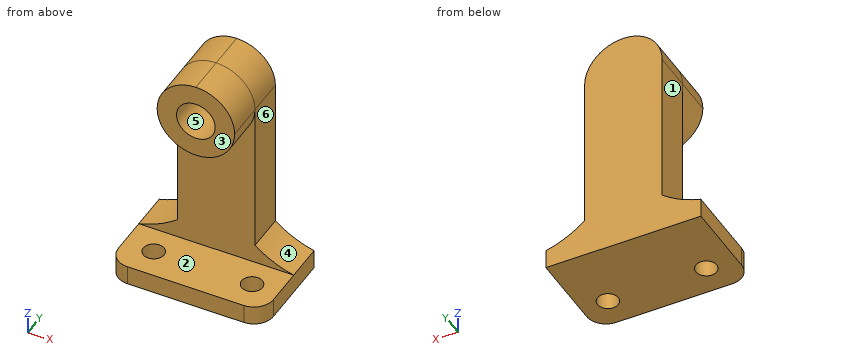
from build123d import *

# Parameters (mm, degrees)
F0_W      = 50.8
F0_H      = 76.2
F1_DEPTH  = 31.75
F2_W      = 19.05
F2_H      = 69.85
F3_DEPTH  = 50.8
F5_DEPTH  = 25.4
F6_R      = 6.35
F7_DEPTH  = 12.7
F8_DEPTH  = 25.4
F9_R      = 3.4236002905
F10_DEPTH = 25.4


with BuildPart() as f1:
    # F0 (on Front) → F1 (new body)
    with BuildSketch(Plane.XZ):
        with Locations((-25.4, 14.5882895922)):
            Rectangle(F0_W, F0_H)
    extrude(amount=F1_DEPTH)

    # F2 (on face) → F3 (cut)
    with BuildSketch(Plane.YZ):
        with Locations((-22.225, 17.7632895922)):
            Rectangle(F2_W, F2_H)
    extrude(amount=-F3_DEPTH, mode=Mode.SUBTRACT)

    # F4 (on face) → F5 (cut)
    with BuildSketch(Plane.XZ.offset(12.7)):
        with BuildLine():
            Line((-50.8, 52.6882895922), (-50.8, -17.1617104078))
            ThreePointArc((-50.8, -17.1617104078), (-44.1071699177, -14.6723705724), (-38.1, -10.8117104078))
            Line((-38.1, -10.8117104078), (-38.1, 52.6882895922))
            Line((-38.1, 52.6882895922), (-50.8, 52.6882895922))
        make_face()
        with BuildLine():
            Line((-12.7, 52.6882895922), (-12.7, -10.8117104078))
            ThreePointArc((-12.7, -10.8117104078), (-6.7122595502, -14.7112295081), (0, -17.1617104078))
            Line((0, -17.1617104078), (0, 52.6882895922))
            Line((0, 52.6882895922), (-12.7, 52.6882895922))
        make_face()
    extrude(amount=-F5_DEPTH, mode=Mode.SUBTRACT)

    # F6 (on face) → F7 (join)
    with BuildSketch(Plane.XZ.offset(12.7)):
        with BuildLine():
            ThreePointArc((-38.1, 39.9882895922), (-25.4, 27.2882895922), (-12.7, 39.9882895922))
            ThreePointArc((-12.7, 39.9882895922), (-16.4197438789, 48.9685457133), (-25.4, 52.6882895922))
            ThreePointArc((-25.4, 52.6882895922), (-34.3802561211, 48.9685457133), (-38.1, 39.9882895922))
        make_face()
        with Locations((-25.4, 39.9882895922)):
            Circle(F6_R, mode=Mode.SUBTRACT)
    extrude(amount=F7_DEPTH)

    # F8 (cut): faces of the model
    f8_faces = [f1.faces().sort_by_distance(p)[0] for p in [
        (-35.2632271754, -12.7, 49.8515167676),
        (-15.5367728246, -12.7, 49.8515167676),
    ]]
    extrude(f8_faces, amount=-F8_DEPTH, mode=Mode.SUBTRACT)

    # F9 (on face) → F10 (cut)
    with BuildSketch(Plane.XY.offset(-17.1617104078)):
        with Locations((-41.0295619067, -21.9763997095)):
            Circle(F9_R)
        with Locations((-8.7823613257, -21.9763997095)):
            Circle(F9_R)
        with BuildLine():
            Line((-50.8, -31.75), (-44.45, -31.75))
            ThreePointArc((-44.45, -31.75), (-48.9401280605, -29.8901280605), (-50.8, -25.4))
            Line((-50.8, -25.4), (-50.8, -31.75))
        make_face()
        with BuildLine():
            ThreePointArc((0, -25.4), (-1.8598719395, -29.8901280605), (-6.35, -31.75))
            Line((-6.35, -31.75), (0, -31.75))
            Line((0, -31.75), (0, -25.4))
        make_face()
    extrude(amount=-F10_DEPTH, mode=Mode.SUBTRACT)


solid = f1.part
Read the model definition and answer for the solid it produces. Units are mm, in the model's axes. Face numbers are marked on the shaded views. A direction names the side the tool comes from. Round coordinates to 2 decimals unless told otherwise and drop trailing zeros. Write each loop counter-clockwise with the first axis right and the second up, starting at its lowest first coordinate (ties: lowest second). Pieces come first, ordered by that corner, then holes.
Q1. Find section C-C on x = -23.5. Determine the outline of the cut face in (y, z), and give its area (3 significant figures).
Values:
outline: (-31.75, -23.51) - (0, -23.51) - (0, 52.55) - (-25.4, 52.55) - (-25.4, 46.05) - (-12.7, 46.05) - (-12.7, 33.93) - (-25.4, 33.93) - (-25.4, 27.43) - (-12.7, 27.43) - (-12.7, -17.16) - (-31.75, -17.16) - close
area: 1,250 mm2
Q2. Find section B-B on y = -23. Determine the outline of the cut face in (x, z), and give its area (3 significant figures).
Values:
outline: (-50.8, -23.51) - (-44.3, -23.51) - (-44.3, -17.16) - (-50.8, -17.16) - close; circle Ø25.4 at (-25.4, 39.99); (-37.76, -23.51) - (-12.05, -23.51) - (-12.05, -17.16) - (-37.76, -17.16) - close; (-5.52, -23.51) - (0, -23.51) - (0, -17.16) - (-5.52, -17.16) - close; hole circle Ø12.7 at (-25.4, 39.99)
area: 620 mm2
Q3. A tool of negligible diameter and unlimited length cuts with its end or side. For the marked faces 1, 2 and 3, from which of +Z, -Z, +X, -X, +Y, -Y can it reach the whole face along a straight path? Write none if from no direction.
Values:
face 1: +Z, -X, +Y, -Y
face 2: +X, -X, -Y
face 3: +Z, +X, -X, -Y
Q4. The mould has two halves that part along Z. Classify the marked faces 4, 5 and 6: released by +Z, released by -Z, zero draft, split by the parting line, or undercut.
Values:
face 4: released by +Z
face 5: undercut
face 6: zero draft
Q5. Flat-ended cylindrical pins translate along their axes: P1, Ø5, axis at y = -4, z = 40, coming from the +X side; P2, Ø3, axis at y = -28.5, z = 27, coming from the +X side; P3, Ø4, axis at x = -28, z = 40.5, coming from the -Y side; P4, Ø6.5, axis at y = -8, z = 14, coming from the -X side. Find the tip coordinate at first contact, or state that the pin passes through.
Values:
P1: stops at x = -12.7
P2: passes through
P3: stops at y = -12.7
P4: stops at x = -38.1
Q6. Find section A-A on y = -14.5. Determine the outline of the cut face in (x, z), and give its area (3 significant figures).
Values:
outline: (-50.8, -23.51) - (0, -23.51) - (0, -17.16) - (-50.8, -17.16) - close; circle Ø25.4 at (-25.4, 39.99); hole circle Ø12.7 at (-25.4, 39.99)
area: 703 mm2
Q7. Straight lines are drawn through the part: line 1 (Z direction, x = -25, y = -21); line 2 (Z direction, x = -25.4, y = -22.5); line 3 (Y direction, x = -14, z = 25.5). For each, find the intervals that lie inside material, in ascending order.
Values:
line 1: z = -23.51 to -17.16, 27.29 to 33.65, 46.33 to 52.68
line 2: z = -23.51 to -17.16, 27.29 to 33.64, 46.34 to 52.69
line 3: y = -12.7 to 0
Q8. Find section D-D on z = 45. Determine the outline of the cut face in (x, y), and give its area (3 significant figures).
Values:
outline: (-37.07, -25.4) - (-29.3, -25.4) - (-29.3, -12.7) - (-21.5, -12.7) - (-21.5, -25.4) - (-13.73, -25.4) - (-13.73, 0) - (-37.07, 0) - close
area: 494 mm2
